The model under review builds one solid part; all positions refer to its coordinate system, in mm. Face numbers are marked on the shaded views. A direction names the side the tool comes from. Round coordinates to 2 decimals unless told otherwise and drop trailing zeros. Loops run counter-clockwise (first coordinate to the right, second up) from the corner with the lowest first, then second, coordinate; pieces in that order, holes last. Notation, with made-up numbers: M 43,89 L 60,89 A21 cw 60,98 Z; hole C 65.25,87 d3. An arc over 180 degrees is marked long. Answer as a JSON object with one key per item and string values. Group by question number.
Item 1: Consider section C-C (y = 0). Give the boundary of the cut face in (x, z).
Item 2: Consider section B-B (x = -43.5). Give the boundary of the cut face in (y, z), and give its area (3 significant figures).
Item 3: Tool access review of the marked faces 1, 2 and 3: name each direction out of +Z, -Z, +X, -X, +Y, -Y from which nothing blocks a thin tool from reaching the whole face with its end or side.
Item 4: Consider section A-A (z = 0). Give the boundary of the cut face in (x, y).
Item 5: To check wall thickness, follow line 1 (Y direction, x = 32.5, z = -22); line 2 (Y direction, x = -54.75, z = 0); line 3 (X direction, y = 47, z = 54). State the ranges of each line that lie inside material, in increasing order.
Item 6: The part is to be moulded in two halves that separate along Y. For the marked faces 4, 5 and 6, say which applies: +Y half, -Y half, draft (parallel to the pull), parting line (faces both ways), or undercut.
Item 7: Consider section D-D (x = 0). Give the boundary of the cut face in (y, z), and give its area (3 significant figures).
Item 8: Insertion check: P1, Ø12, axis at x = 27.5, z = -43.5, coming from the +Y side; P2, Ø3, axis at y = -27, z = 17, coming from the +X side; P3, Ø6, axis at x = -15, z = 1.5, coming from the +Y side. Each pin has a flat end and moves straight along its axis. Give the tip position at first contact, or say it passes through.
```python
from build123d import *

# Parameters (mm, degrees)
SWEEP1_PROFILE_R    = 10
CUT_EXTRUDE1_START  = -5.9
SKETCH13_R          = 10
CUT_EXTRUDE1_DEPTH  = 5.9
SKETCH14_R          = 10
BOSS_EXTRUDE1_DEPTH = 4
BOSS_EXTRUDE2_DEPTH = 10
BOSS_EXTRUDE3_DEPTH = 120
SKETCH18_W          = 120
SKETCH18_H          = 142
CUT_EXTRUDE2_DEPTH  = 203.932082269
SKETCH19_R          = 30
CUT_EXTRUDE3_DEPTH  = 18
FILLET1_R           = 10


with BuildPart() as part:
    # Sweep1: sweep along a path in Sketch2
    with BuildLine(Plane(origin=(0, 0, 0), x_dir=(0, 0, -1), z_dir=(1, 0, 0))) as sweep1_path:
        Line((0, 158.93373393), (0, -158.93373393))
    # Sweep1 profile (on start of the path) → Sweep1 (sweep)
    with BuildSketch(Plane(origin=(0, 158.93373393, 0), x_dir=(0, 0, -1), z_dir=(0, -1, 0))):
        Circle(SWEEP1_PROFILE_R)
    sweep(path=sweep1_path.line)

    # Sketch13 → Cut-Extrude1 (cut)
    with BuildSketch(Plane(origin=(0, 158.93373393, 0), x_dir=(1, 0, 0), z_dir=(0, 1, 0)).offset(CUT_EXTRUDE1_START)):
        with Locations(Location((0, 0, 0), (0, 0, 90))):
            Circle(SKETCH13_R)
    extrude(amount=CUT_EXTRUDE1_DEPTH, mode=Mode.SUBTRACT)

    # Sketch14 → Boss-Extrude1 (add)
    with BuildSketch(Plane(origin=(0, 153.03373393, 0), x_dir=(1, 0, 0), z_dir=(0, 1, 0))):
        with Locations(Location((0, 0, 0), (0, 0, 90))):
            Circle(SKETCH14_R)
    extrude(amount=BOSS_EXTRUDE1_DEPTH)

    # Sketch16 → Boss-Extrude2 (add)
    with BuildSketch(Plane(origin=(0, 80.05, 0), x_dir=(-1, 0, 0), z_dir=(0, -1, 0))):
        with BuildLine():
            Line((11.012438692, 60), (60, 60))
            Line((60, 60), (60, -60))
            Line((60, -60), (11.012438692, -60))
            Line((11.012438692, -60), (-11.012438692, -60))
            ThreePointArc((-11.012438692, -60), (-61.00224427, 0), (-11.012438692, 60))
            Line((-11.012438692, 60), (11.012438692, 60))
        make_face()
    boss_extrude2 = extrude(amount=BOSS_EXTRUDE2_DEPTH)

    # Mirror1: Boss-Extrude2 across plane
    add(boss_extrude2.mirror(Plane(origin=(0, -0.95, 0), x_dir=(0, 0, 1), z_dir=(0, -1, 0))))

    # Sketch17 → Boss-Extrude3 (add)
    with BuildSketch(Plane(origin=(0, 0, -60), x_dir=(-1, 0, 0), z_dir=(0, 0, -1))):
        Polygon((60, -71.95), (50, -71.95), (50, 70.05), (60, 70.05), (60, 80.05), (68, 80.05), (68, -81.95), (60, -81.95), align=None)
    extrude(amount=-BOSS_EXTRUDE3_DEPTH)

    # Sketch18 → Cut-Extrude2 (cut, through all)
    with BuildSketch(Plane(origin=(-50, 0, 0), x_dir=(0, 0, -1), z_dir=(1, 0, 0))):
        with Locations((0, -0.95)):
            Rectangle(SKETCH18_W, SKETCH18_H)
    extrude(amount=CUT_EXTRUDE2_DEPTH, mode=Mode.SUBTRACT)

    # Sketch19 → Cut-Extrude3 (cut)
    with BuildSketch(Plane.ZY.offset(68)):
        Circle(SKETCH19_R)
    extrude(amount=-CUT_EXTRUDE3_DEPTH, mode=Mode.SUBTRACT)

    # Fillet1
    fillet1_edges = [part.edges().sort_by_distance(p)[0] for p in [
        (0, 80.05, 10),
        (0, -81.95, 10),
        (-68, 80.05, 0),
        (-68, -81.95, 0),
    ]]
    fillet(fillet1_edges, radius=FILLET1_R)


solid = part.part
```
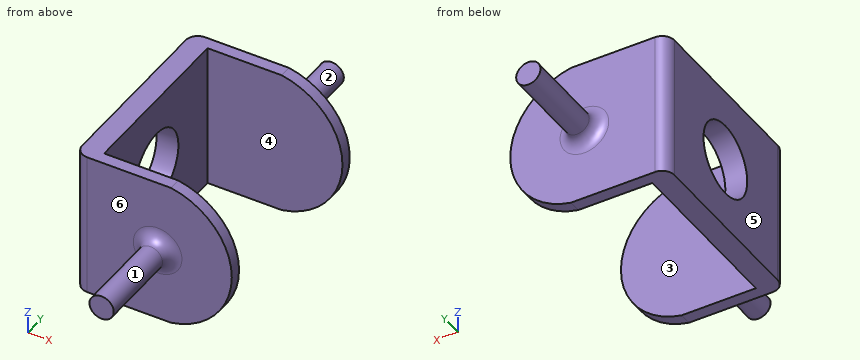
Geometry results:
{
 "1": {"outline": "M -68,-60 L -50,-60 L -50,-30 L -68,-30 Z; M -68,30 L -50,30 L -50,60 L -68,60 Z"},
 "2": {"outline": "M -81.95,-60 L -71.95,-60 L -71.95,60 L -81.95,60 Z; M 70.05,-60 L 80.05,-60 L 80.05,60 L 70.05,60 Z", "area": "2,400 mm^2"},
 "3": {"face 1": "-Y", "face 2": "+Y", "face 3": "+Z, -Z, +X"},
 "4": {"outline": "M -68,-71.95 A10 ccw -58,-81.95 L -20,-81.95 A10 cw -10,-91.95 L -10,-158.93 L 10,-158.93 L 10,-91.95 A10 cw 20,-81.95 L 61,-81.95 L 61,-71.95 L -50,-71.95 L -50,-30 L -68,-30 Z; M -68,30 L -50,30 L -50,70.05 L 61,70.05 L 61,80.05 L 20,80.05 A10 cw 10,90.05 L 10,157.03 L -10,157.03 L -10,90.05 A10 cw -20,80.05 L -58,80.05 A10 ccw -68,70.05 Z"},
 "5": {"line 1": "y = -81.95 to -71.95, 70.05 to 80.05", "line 2": "y = -81.95 to -30, 30 to 80.05", "line 3": "x = -68 to -50"},
 "6": {"face 4": "undercut", "face 5": "draft", "face 6": "-Y half"},
 "7": {"outline": "M -158.93,-10 L -91.95,-10 A10 cw -81.95,-20 L -81.95,-60 L -71.95,-60 L -71.95,60 L -81.95,60 L -81.95,20 A10 cw -91.95,10 L -158.93,10 Z; M 70.05,-60 L 80.05,-60 L 80.05,-20 A10 cw 90.05,-10 L 157.03,-10 L 157.03,10 L 90.05,10 A10 cw 80.05,20 L 80.05,60 L 70.05,60 Z", "area": "5,570 mm^2"},
 "8": {"P1": "stops at y = 80.05", "P2": "stops at x = -50", "P3": "stops at y = 83.95"}
}
